Read the model definition and answer for the solid it produces. Units are mm, in the model's axes. Face numbers are marked on the shaded views. A direction names the side the tool comes from. Coordinates: 2 decimals unless noted, no trailing zeros. Write each loop counter-clockwise with the first axis right and the second up, starting at its lowest first coordinate (ties: lowest second). Pieces come first, ordered by that corner, then holes.
(1) The mould has two halves that part along Y. Classify the marked faces 5, 6 and 7: +Y half, -Y half, draft (parallel to the pull), parting line (faces both ways), or undercut.
(2) Find the intervals of material crossed by probe 1 along Y at (x, z) = (0, 8.25); probe 2 along X at (y, z) = (-5, 9.25); probe 3 along X at (y, z) = (-25, 1.5), in increasing order.
(3) Section D-D on z = 7.25 is taken. State how many separate pieces and enclosed holes the cut face has, then the cut area to 3 significant figures.
(4) Section A-A on x = 0 is taken. Write down the section's boundary in (y, z), then the cut area to 3 significant figures.
(5) Which of the six approach directions +Z, -Z, +X, -X, +Y, -Y give full straight-line access (tool end or side, diameter ignored) to the marked faces 1, 2, 3 and 4?
(6) Section C-C on y = 20 is taken. Write down the section's boundary in (x, z).
(7) Given pin 1 (6 mm diameter, centred on y = 5.5, z = 5.5, fed in from +X); pin 2 (3 mm diameter, centred on y = 7, z = 3.5, fed in from -X); pin 3 (4.5 mm diameter, centred on x = -21.21, y = -21.21, fed in from -Z); pin 4 (6 mm diameter, centred on y = 12.5, z = 6, fed in from +X), each flat-ended and moving along its own axis, determine where each tip first touches the part or whether it passes through.
from build123d import *

# Parameters (mm, degrees)
SKETCH1_R           = 2.5
SKETCH1_R_2         = 7.5
BOSS_EXTRUDE1_DEPTH = 10


with BuildPart() as part:
    # Sketch1 → Boss-Extrude1 (new body)
    with BuildSketch(Plane.XY):
        with BuildLine():
            Line((17.928932188, 30), (25, 30))
            ThreePointArc((25, 30), (28.535533906, 28.535533906), (30, 25))
            Line((30, 25), (30, 17.928932188))
            ThreePointArc((30, 17.928932188), (29.619397663, 16.015515026), (28.535533906, 14.393398282))
            Line((28.535533906, 14.393398282), (17.67766953, 3.535533906))
            ThreePointArc((17.67766953, 3.535533906), (16.213203436, 0), (17.67766953, -3.535533906))
            Line((17.67766953, -3.535533906), (28.535533906, -14.393398282))
            ThreePointArc((28.535533906, -14.393398282), (29.619397663, -16.015515026), (30, -17.928932188))
            Line((30, -17.928932188), (30, -25))
            ThreePointArc((30, -25), (28.535533906, -28.535533906), (25, -30))
            Line((25, -30), (17.928932188, -30))
            ThreePointArc((17.928932188, -30), (16.015515026, -29.619397663), (14.393398282, -28.535533906))
            Line((14.393398282, -28.535533906), (3.535533906, -17.67766953))
            ThreePointArc((3.535533906, -17.67766953), (0, -16.213203436), (-3.535533906, -17.67766953))
            Line((-3.535533906, -17.67766953), (-14.393398282, -28.535533906))
            ThreePointArc((-14.393398282, -28.535533906), (-16.015515026, -29.619397663), (-17.928932188, -30))
            Line((-17.928932188, -30), (-25, -30))
            ThreePointArc((-25, -30), (-28.535533906, -28.535533906), (-30, -25))
            Line((-30, -25), (-30, -17.928932188))
            ThreePointArc((-30, -17.928932188), (-29.619397663, -16.015515026), (-28.535533906, -14.393398282))
            Line((-28.535533906, -14.393398282), (-17.67766953, -3.535533906))
            ThreePointArc((-17.67766953, -3.535533906), (-16.213203436, 0), (-17.67766953, 3.535533906))
            Line((-17.67766953, 3.535533906), (-28.535533906, 14.393398282))
            ThreePointArc((-28.535533906, 14.393398282), (-29.619397663, 16.015515026), (-30, 17.928932188))
            Line((-30, 17.928932188), (-30, 25))
            ThreePointArc((-30, 25), (-28.535533906, 28.535533906), (-25, 30))
            Line((-25, 30), (-17.928932188, 30))
            ThreePointArc((-17.928932188, 30), (-16.015515026, 29.619397663), (-14.393398282, 28.535533906))
            Line((-14.393398282, 28.535533906), (-3.535533906, 17.67766953))
            ThreePointArc((-3.535533906, 17.67766953), (0, 16.213203436), (3.535533906, 17.67766953))
            Line((3.535533906, 17.67766953), (14.393398282, 28.535533906))
            ThreePointArc((14.393398282, 28.535533906), (16.015515026, 29.619397663), (17.928932188, 30))
        make_face()
        with Locations((-21.213203436, 21.213203436)):
            Circle(SKETCH1_R, mode=Mode.SUBTRACT)
        with Locations((21.213203436, 21.213203436)):
            Circle(SKETCH1_R, mode=Mode.SUBTRACT)
        with Locations((21.213203436, -21.213203436)):
            Circle(SKETCH1_R, mode=Mode.SUBTRACT)
        with Locations((-21.213203436, -21.213203436)):
            Circle(SKETCH1_R, mode=Mode.SUBTRACT)
        Circle(SKETCH1_R_2, mode=Mode.SUBTRACT)
    extrude(amount=BOSS_EXTRUDE1_DEPTH)


solid = part.part
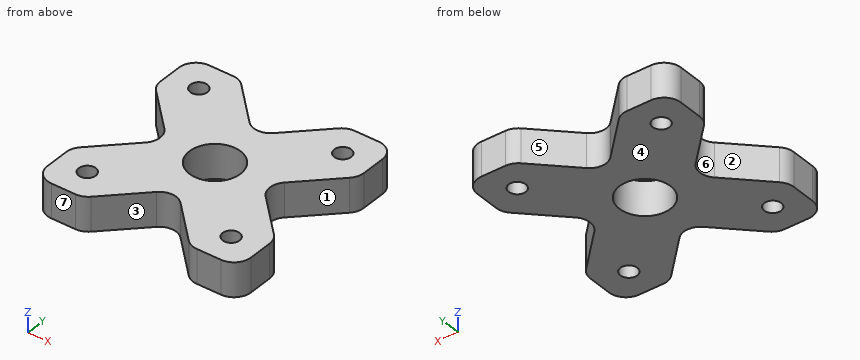
Response:
1. face 5: +Y half
1. face 6: undercut
1. face 7: -Y half
2. probe 1: y = -16.21 to -7.5, 7.5 to 16.21
2. probe 2: x = -19.14 to -5.59, 5.59 to 19.14
2. probe 3: x = -30 to -10.86, 10.86 to 30
3. separate pieces: 1
3. enclosed holes: 5
3. area: 2,330 mm2
4. outline: (-16.21, 0) - (-7.5, 0) - (-7.5, 10) - (-16.21, 10) - close; (7.5, 0) - (16.21, 0) - (16.21, 10) - (7.5, 10) - close
4. area: 174 mm2
5. face 1: +Z, -Z, +X
5. face 2: +Z, -Z, -X
5. face 3: +Z, -Z, -Y
5. face 4: -Z, +X, -X, +Y, -Y
6. outline: (-30, 0) - (-23.4, 0) - (-23.4, 10) - (-30, 10) - close; (-19.03, 0) - (-5.86, 0) - (-5.86, 10) - (-19.03, 10) - close; (5.86, 0) - (19.03, 0) - (19.03, 10) - (5.86, 10) - close; (23.4, 0) - (30, 0) - (30, 10) - (23.4, 10) - close
7. pin 1: stops at x = 22.64
7. pin 2: stops at x = -22.64
7. pin 3: passes through
7. pin 4: stops at x = 29.37
